The listing builds one solid part. Answer for the finished solid, in the listing's coordinates (mm). A direction names the side the tool comes from. Round coordinates to 2 decimals unless told otherwise and drop trailing zeros. Write each loop counter-clockwise with the first axis right and the second up, starting at its lowest first coordinate (ties: lowest second). Pieces come first, ordered by that corner, then holes. Notation, with made-up numbers: (-37.5, -25.5) - (-23.5, -25.5) arc R23 ccw to (-23.5, -6.5) - close; hole circle Ø1 at (80, 64). An arc over 180 degrees is marked (long way). Return JSON: item names as keys, results as strings. Group by question number.
from build123d import *

# Parameters (mm, degrees)
SKETCH1_R           = 2
BOSS_EXTRUDE1_DEPTH = 2
SKETCH2_R           = 1.6
CUT_EXTRUDE1_DEPTH  = 10
CHAMFER1_SIZE       = 2


with BuildPart() as part:
    # Sketch1 → Boss-Extrude1 (new body)
    with BuildSketch(Plane(origin=(0, 50.662802213, 0), x_dir=(1, 0, 0), z_dir=(0, 1, 0))):
        Polygon((-85.703232371, -20), (-85.703232371, -40), (-96.203232371, -40), (-96.203232371, -116), (-85.703232371, -116), (-85.703232371, -136), (-51.703232371, -136), (-51.703232371, -116), (-41.203232371, -116), (-41.203232371, -40), (-51.703232371, -40), (-51.703232371, -20), align=None)
        with Locations((-79.703232371, -30)):
            Circle(SKETCH1_R, mode=Mode.SUBTRACT)
        with Locations((-79.703232371, -126)):
            Circle(SKETCH1_R, mode=Mode.SUBTRACT)
        with Locations((-57.703232371, -126)):
            Circle(SKETCH1_R, mode=Mode.SUBTRACT)
    extrude(amount=BOSS_EXTRUDE1_DEPTH)

    # Sketch2 → Cut-Extrude1 (cut)
    with BuildSketch(Plane(origin=(0, 52.662802213, 0), x_dir=(1, 0, 0), z_dir=(0, 1, 0))):
        with Locations((-92.903232371, -54)):
            Circle(SKETCH2_R)
        with Locations((-44.503232371, -55.2)):
            Circle(SKETCH2_R)
        with Locations((-89.403232371, -106)):
            Circle(SKETCH2_R)
        with Locations((-61.403232371, -106)):
            Circle(SKETCH2_R)
    extrude(amount=-CUT_EXTRUDE1_DEPTH, mode=Mode.SUBTRACT)

    # Chamfer1
    chamfer1_edges = [part.edges().sort_by_distance(p)[0] for p in [
        (-51.703232371, 51.662802213, 20),
        (-41.203232371, 51.662802213, 40),
        (-41.203232371, 51.662802213, 116),
        (-51.703232371, 51.662802213, 136),
        (-85.703232371, 51.662802213, 136),
        (-96.203232371, 51.662802213, 116),
        (-96.203232371, 51.662802213, 40),
        (-85.703232371, 51.662802213, 20),
    ]]
    chamfer(chamfer1_edges, length=CHAMFER1_SIZE)


solid = part.part
(1) Determine the mould class of faces 4 (the cylindrical face through (-77.856, 51.649, 30.766)), 5 (the flat face through (-69, 52.663, 77)), 6 (the cylindrical face through (-45.682, 51.677, 54.119)), 7 (the flat face through (-52.689, 51.649, 21.014)) for opening direction X: +X half, -X half, draft (parallel to the pull), parting line (faces both ways), or undercut.
(2) Find section C-C (x = -45). Write down the section's boundary in (y, z), plus the area to 3 significant figures.
(3) Find section B-B (y = 51.2). Write down the section's boundary in (x, z), plus the area to 3 significant figures.
(4) For faces 1 (the flat face through (-47, 52, 40)), 2 (the flat face through (-51.703, 52, 125)), 3 (the flat face through (-85.703, 52, 31)), determine the directions among +Z, -Z, +X, -X, +Y, -Y from which every point of the face is accessible in a straight line to the end or side of a thin tool.
(5) Find section A-A (z = 126). Write down the section's boundary in (x, y), plus the area to 3 significant figures.
(6) Consider line 1 (X direction, y = 51.4, z = 126); line 2 (X direction, y = 51.55, z = 106); line 3 (Z direction, x = -80.5, y = 51.6). Determine where each line is inside the solid, lowest interval first.
(7) Flat-ended cylindrical pins translate along their axes: pin 1 (0.6 mm diameter, centred on y = 52, z = 31.5, fed in from -X); pin 2 (4.5 mm diameter, centred on x = -57.7, z = 126, fed in from -Y); pin 3 (0.6 mm diameter, centred on x = -46.5, y = 52, fed in from -Z); pin 4 (1 mm diameter, centred on x = -89, y = 52, fed in from +Z). Find the tip coordinate at first contact, or state that the pin passes through.
(8) Find section D-D (z = 106). Write down the section's boundary in (x, y).
Check sheet entries:
{
 "1": {"face 4": "undercut", "face 5": "draft", "face 6": "undercut", "face 7": "+X half"},
 "2": {"outline": "(50.66, 40) - (52.66, 40) - (52.66, 53.68) - (50.66, 53.68) - close; (50.66, 56.72) - (52.66, 56.72) - (52.66, 116) - (50.66, 116) - close", "area": "146 mm^2"},
 "3": {"outline": "(-96.2, 42) - (-94.2, 40) - (-85.7, 40) - (-85.7, 22) - (-83.7, 20) - (-53.7, 20) - (-51.7, 22) - (-51.7, 40) - (-43.2, 40) - (-41.2, 42) - (-41.2, 114) - (-43.2, 116) - (-51.7, 116) - (-51.7, 134) - (-53.7, 136) - (-83.7, 136) - (-85.7, 134) - (-85.7, 116) - (-94.2, 116) - (-96.2, 114) - close; hole circle Ø3.2 at (-92.9, 54); hole circle Ø3.2 at (-89.4, 106); hole circle Ø4 at (-79.7, 30); hole circle Ø4 at (-79.7, 126); hole circle Ø3.2 at (-61.4, 106); hole circle Ø4 at (-57.7, 126); hole circle Ø3.2 at (-44.5, 55.2)", "area": "5,450 mm^2"},
 "4": {"face 1": "-Z, +X, +Y, -Y", "face 2": "+Z, +X, +Y, -Y", "face 3": "-Z, -X, +Y, -Y"},
 "5": {"outline": "(-85.7, 50.66) - (-81.7, 50.66) - (-81.7, 52.66) - (-85.7, 52.66) - close; (-77.7, 50.66) - (-59.7, 50.66) - (-59.7, 52.66) - (-77.7, 52.66) - close; (-55.7, 50.66) - (-51.7, 50.66) - (-51.7, 52.66) - (-55.7, 52.66) - close", "area": "52.0 mm^2"},
 "6": {"line 1": "x = -85.7 to -81.7, -77.7 to -59.7, -55.7 to -51.7", "line 2": "x = -96.2 to -91, -87.8 to -63, -59.8 to -41.2", "line 3": "z = 20 to 28.17, 31.83 to 124.17, 127.83 to 136"},
 "7": {"pin 1": "stops at x = -85.7", "pin 2": "stops at y = 50.66", "pin 3": "stops at z = 40", "pin 4": "stops at z = 116"},
 "8": {"outline": "(-96.2, 50.66) - (-91, 50.66) - (-91, 52.66) - (-96.2, 52.66) - close; (-87.8, 50.66) - (-63, 50.66) - (-63, 52.66) - (-87.8, 52.66) - close; (-59.8, 50.66) - (-41.2, 50.66) - (-41.2, 52.66) - (-59.8, 52.66) - close"}
}
